Autodesk Inventor part; units mm, degrees
ref_plane "YZ Plane" through (0, 0, 0) normal (1, 0, 0) x (0, 1, 0)
ref_plane "XZ Plane" through (0, 0, 0) normal (0, 1, 0) x (-1, 0, 0)
ref_plane "XY Plane" through (0, 0, 0) normal (0, 0, 1) x (1, 0, 0)
sketch "Sketch1" plane through (0, 0, 0) normal (0, 0, 1) x (1, 0, 0)
  line L0 (-60, -45) -> (60, -45)
  line L1 (60, -45) -> (60, 45)
  line L2 (60, 45) -> (-60, 45)
  line L3 (-60, 45) -> (-60, -45)
  line L4 (-60, -45) -> (60, 45) construction
  line L5 (60, -45) -> (-60, 45) construction
  line L6 (-50, -35) -> (50, -35)
  line L7 (50, -35) -> (50, 35)
  line L8 (50, 35) -> (-50, 35)
  line L9 (-50, 35) -> (-50, -35)
  line L10 (-50, -35) -> (50, 35) construction
  line L11 (50, -35) -> (-50, 35) construction
  point P0 (0, 0)
  dimension "d0" = 120
  dimension "d1" = 90
  dimension "d2" = 100
  dimension "d3" = 70
extrude "Extrusion1" add sketch "Sketch1" along normal blind 6
sketch "Sketch2" plane through (60, -45, 0) normal (1, 0, 0) x (0, 0, -1)
  line L0 (0, 0) -> (0, 90)
  line L1 (0, 90) -> (-6, 90)
  line L2 (-6, 0) -> (-6, 90)
  line L3 (0, 0) -> (-6, 0)
  line L4 (0, 45) -> (-3, 45)
  line L5 (-3.6, 9.9) -> (-2.4, 9.9)
  line L6 (-2.4, 9.9) -> (-2.4, 80.1)
  line L7 (-2.4, 80.1) -> (-3.6, 80.1)
  line L8 (-3.6, 80.1) -> (-3.6, 9.9)
  line L9 (-3.6, 9.9) -> (-2.4, 80.1) construction
  line L10 (-2.4, 9.9) -> (-3.6, 80.1) construction
  dimension "d6" = 3
  dimension "d7" = 1.2
  dimension "d8" = 70.2
extrude "Extrusion2" cut sketch "Sketch2" against normal blind 120 contours L6 L5 L8 L7
sketch "Sketch3" plane through (-60, -45, 0) normal (0, -1, 0) x (1, 0, 0)
  line L0 (60, 0) -> (60, 3)
  line L1 (120, 33) -> (0, 33)
  line L2 (0, 33) -> (0, -27)
  line L3 (0, -27) -> (120, -27)
  line L4 (120, -27) -> (120, 33)
  line L5 (120, 33) -> (0, -27) construction
  line L6 (0, 33) -> (120, -27) construction
  dimension "d11" = 3
  dimension "d12" = 120
  dimension "d13" = 60
extrude "Extrusion3" add sketch "Sketch3" against normal blind 3
fillet "Fillet1" radius 4 2 edges at (0, -42, 6) (0, -42, 0)
fillet "Fillet2" radius 6 2 edges at (-60, 45, 3) (60, 45, 3)
fillet "Fillet3" radius 10 4 edges at (60, -43.5, 33) (60, -43.5, -27) (-60, -43.5, 33) (-60, -43.5, -27)
equation "\"d0\" = tot_w"
equation "\"d1\" = tot_h"
equation "\"d2\" = window_width"
equation "\"d3\" = window_height"
equation "\"d4\" = tot_t"
equation "\"d6\" = 0.5 * tot_t"
equation "\"d7\" = t + 2 * offset"
equation "\"d8\" = window_height + 2 * offset"
equation "\"d9\" = tot_w"
equation "\"d11\" = 0.5 * tot_t"
equation "\"d12\" = tot_w"
equation "\"d13\" = base_w"
equation "\"window_width\" = 100"
equation "\"window_height\" = 70"
equation "\"t\" = 1"
equation "\"offset\" = 0.1"
equation "\"tot_t\" = 6"
equation "\"tot_w\" = 120"
equation "\"tot_h\" = 90"
equation "\"base_w\" = 60"
properties part number "light_frame_v1"
Work out the finished part from the listing and answer in its coordinate system (mm). A direction names the side the tool comes from. Give positions to 0.01 mm unless a question says otherwise; leave off trailing zeros. Order: outer loops, then holes, each group sorted by start corner. A loop starts at its lowest first (then second) coordinate and runs counter-clockwise, first axis right, second up. Notation, with made-up numbers: M 72,89 L 84,89 A17 ccw 84,101 Z; hole C -19,86 d7. An arc over 180 degrees is marked long. Return JSON: item names as keys, results as strings.
1) Section A-A, the plane y = 22 is taken. Write down the section's boundary in (x, z).
Resolved:
{"outline": "M -60,0 L -50,0 L -50,2.4 L -60,2.4 Z; M -60,3.6 L -50,3.6 L -50,6 L -60,6 Z; M 50,0 L 60,0 L 60,2.4 L 50,2.4 Z; M 50,3.6 L 60,3.6 L 60,6 L 50,6 Z"}
2) For a pull along Y with two mould halves and no side action, classify faces 1 (the flat face through (4, 38, 0)), 2 (the cylindrical face through (-58.196, 43.289, 3.042)), 3 (the flat face through (-53, -3, 2.4)) as +Y half, -Y half, draft (parallel to the pull), parting line (faces both ways), or undercut.
Resolved:
{"face 1": "draft", "face 2": "+Y half", "face 3": "undercut"}
3) This flat-tipped pin is pushed along its axis until it touches: pin 1 (7 mm diameter, centred on x = 25, z = 25, fed in from +Y). Where does it stop, or does it pass through?
Resolved:
{"pin 1": "y = -42"}
4) Straight lines are drawn through the part: line 1 along Y through (x, z) = (36, 1.5); line 2 along X through (y, z) = (19, 1.5); line 3 along Z through (x, y) = (-51, 34.5). For each, find the intervals that lie inside material, in ascending order. Write a range as [from, to].
Resolved:
{"line 1": "[-45, -35], [35, 45]", "line 2": "[-60, -50], [50, 60]", "line 3": "[0, 2.4], [3.6, 6]"}
5) Section D-D, the plane z = 27 is taken. Write down the section's boundary in (x, y).
Resolved:
{"outline": "M -59.17,-45 L 59.17,-45 L 59.17,-42 L -59.17,-42 Z"}
6) A tool of negligible diameter and unlimited length cuts with its end or side. For faces 4 (the flat face through (-53, 3, 3.6)), 5 (the flat face through (4, 38, 6)), 6 (the flat face through (-1, -42, -15)), from which of +Z, -Z, +X, -X, +Y, -Y can it reach the whole face along a straight path? Write none if from no direction.
Resolved:
{"face 4": "+X, -X", "face 5": "+Z, +X, -X, +Y", "face 6": "-Z, +X, -X, +Y"}
7) Section C-C, the plane z = -13.5 is taken. Write down the section's boundary in (x, y), plus the area to 3 significant figures.
Resolved:
{"outline": "M -60,-45 L 60,-45 L 60,-42 L -60,-42 Z", "area": "360 mm^2"}
8) Section B-B, the plane x = -3 is taken. Write down the section's boundary in (y, z).
Resolved:
{"outline": "M -45,-27 L -42,-27 L -42,-4 A4 cw -38,0 L -35,0 L -35,2.4 L -35.1,2.4 L -35.1,3.6 L -35,3.6 L -35,6 L -38,6 A4 cw -42,10 L -42,33 L -45,33 Z; M 35,0 L 45,0 L 45,6 L 35,6 L 35,3.6 L 35.1,3.6 L 35.1,2.4 L 35,2.4 Z"}
